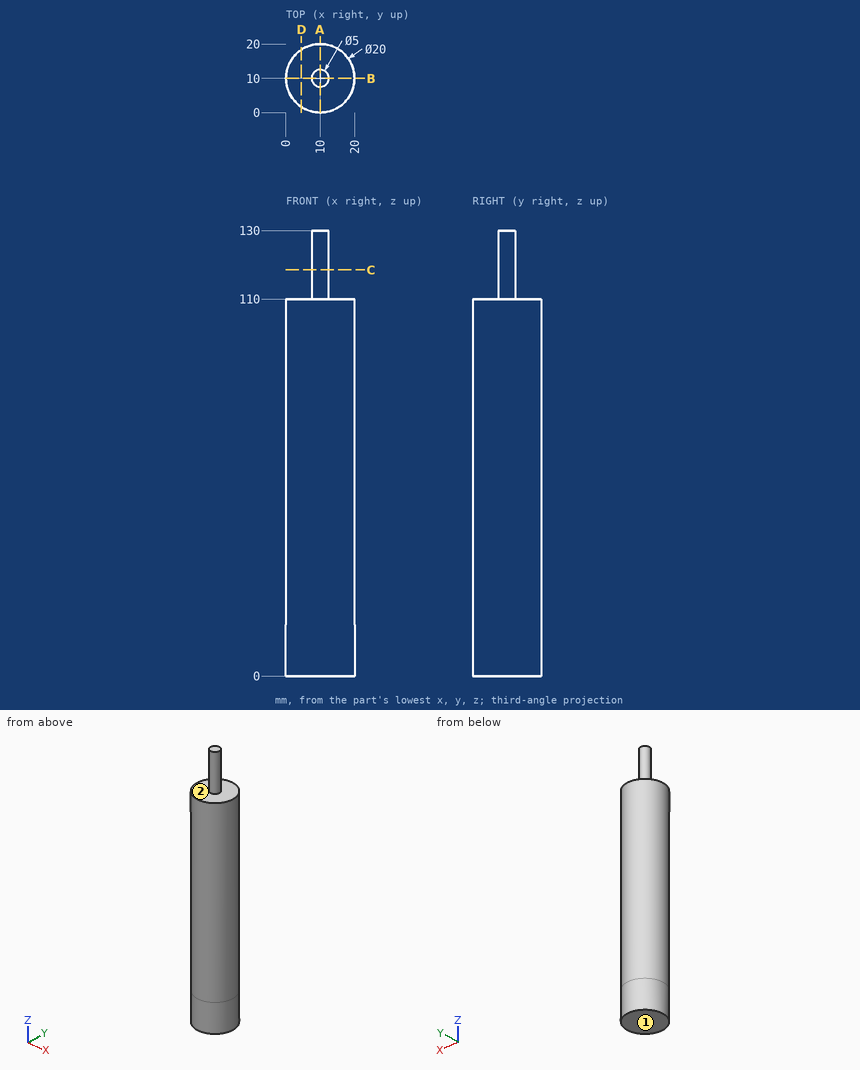
Here's the drawing with two shaded views (mm, measured from the low corner). I have some questions. A direction names the side the tool comes from. Coordinates: 2 decimals unless noted, no trailing zeros. Write each loop counter-clockwise with the first axis right and the second up, starting at its lowest first coordinate (ties: lowest second). Pieces come first, ordered by that corner, then holes. Notation, with made-up numbers: (79, 60) -> (85, 60) arc R19 ccw to (85, 87) -> close; hole circle Ø4 at (29.25, 67). An arc over 180 degrees is marked (long way). Write item = value, one per line. Start each with the question number.
(1) Will these pins go through, and if not, where does the flat tip stop? pin 1 (4 mm diameter, centred on y = 3, z = 60.5, fed in from -X); pin 2 (3 mm diameter, centred on y = 13, z = 79, fed in from -X); pin 3 (8 mm diameter, centred on x = 16.5, z = 31.5, fed in from +Y); pin 4 (10 mm diameter, centred on x = 12.5, y = 2, fed in from -Z).
(2) I want a section at D-D (x = 4.5). Please give me the cut outline in (y, z), plus the area to 3 significant figures.
(3) I want a section at A-A (x = 10). Please give me the cut outline in (y, z), plus the area to 3 significant figures.
(4) I need wall thicknesses on line 1 (Z direction, x = 1.75, y = 14.75); line 2 (Y direction, x = 9.5, z = 94.5); line 3 (X direction, y = 10.25, z = 7.5). Which ranges of each line are inside material? Lowest first, please. Write a range as [from, to].
(5) I want a section at C-C (z = 118.5). Please give me the cut outline in (x, y).
(6) Which directions (+Z, -Z, +X, -X, +Y, -Y) give clear straight access to the entire face, cutting with the end or side of a thin tool? Please do the marked faces 1 and 2.
Result set:
q1.pin_1 = 1.34
q1.pin_2 = 0.11
q1.pin_3 = 19.68
q1.pin_4 = 0
q2.outline = (1.65, 0) -> (18.35, 0) -> (18.35, 110) -> (1.65, 110) -> close
q2.area = 1,840 mm2
q3.outline = (0, 0) -> (20, 0) -> (20, 110) -> (12.5, 110) -> (12.5, 130) -> (7.5, 130) -> (7.5, 110) -> (0, 110) -> close
q3.area = 2,300 mm2
q4.line_1 = [0, 110]
q4.line_2 = [0.01, 19.99]
q4.line_3 = [0, 20]
q5.outline = circle Ø5 at (10, 10)
q6.face_1 = -Z, +X, -X, +Y, -Y
q6.face_2 = +Z
